Geometry check sheet. Reference: the model listing, model coordinates, mm. A direction names the side the tool comes from. Coordinates: 2 decimals unless noted, no trailing zeros. Write each loop counter-clockwise with the first axis right and the second up, starting at its lowest first coordinate (ties: lowest second). Pieces come first, ordered by that corner, then holes. Notation, with made-up numbers: (64, 83) -> (100, 83) arc R13 ccw to (100, 100) -> close; hole circle Ø10 at (68, -7). An arc over 180 degrees is marked (long way). Put each result on its own line as item: value. Start each with the question number.
from build123d import *

# Parameters (mm, degrees)
SKETCH_1_W          = 280
SKETCH_1_H          = 230
EXTRUDE_1_DEPTH     = 2
SKETCH_2_R          = 2.15
CUT_EXTRUDE_1_DEPTH = 182.18774793
SKETCH_3_R          = 30
CUT_EXTRUDE_2_DEPTH = 182.18774793
SKETCH_4_R          = 1.6
CUT_EXTRUDE_3_DEPTH = 182.18774793
SKETCH_5_R          = 1.65
CUT_EXTRUDE_4_DEPTH = 182.18774793
SKETCH_7_W          = 25
SKETCH_7_H          = 115
SKETCH_7_W_2        = 85
SKETCH_7_H_2        = 15
CUT_EXTRUDE_5_DEPTH = 182.18774793
SKETCH_9_W          = 36
SKETCH_9_H          = 17
CUT_EXTRUDE_6_DEPTH = 182.18774793
FILLET_1_R          = 2
FILLET_2_R          = 2


with BuildPart() as part:
    # 草图1 → 凸台-拉伸1 (new body)
    with BuildSketch(Plane.XY):
        Rectangle(SKETCH_1_W, SKETCH_1_H)
    extrude(amount=EXTRUDE_1_DEPTH)

    # 草图2 → 切除-拉伸1 (cut, through all)
    with BuildSketch(Plane.XY.offset(2)):
        with Locations((-132.5, -105)):
            Circle(SKETCH_2_R)
        with Locations(Location((132.5, -105, 0), (0, 0, 180))):
            Circle(SKETCH_2_R)
        with Locations((-115, -87.5)):
            Circle(SKETCH_2_R)
        with Locations((-95, -87.5)):
            Circle(SKETCH_2_R)
        with Locations((-75, -87.5)):
            Circle(SKETCH_2_R)
        with Locations(Location((75, -87.5, 0), (0, 0, 180))):
            Circle(SKETCH_2_R)
        with Locations(Location((95, -87.5, 0), (0, 0, 180))):
            Circle(SKETCH_2_R)
        with Locations(Location((115, -87.5, 0), (0, 0, 180))):
            Circle(SKETCH_2_R)
    extrude(amount=-CUT_EXTRUDE_1_DEPTH, mode=Mode.SUBTRACT)

    # 草图3 → 切除-拉伸2 (cut, through all)
    with BuildSketch(Plane.XY.offset(2)):
        with Locations((0, -5)):
            Circle(SKETCH_3_R)
        with BuildLine():
            ThreePointArc((30, -5), (0, -35), (-30, -5))
            Line((-30, -5), (-30, -115))
            Line((-30, -115), (30, -115))
            Line((30, -115), (30, -5))
        make_face()
    extrude(amount=-CUT_EXTRUDE_2_DEPTH, mode=Mode.SUBTRACT)

    # 草图4 → 切除-拉伸3 (cut, through all)
    with BuildSketch(Plane.XY.offset(2)):
        with Locations((-109, -35)):
            Circle(SKETCH_4_R)
        with Locations((-109, -55)):
            Circle(SKETCH_4_R)
        with Locations((-116, -35)):
            Circle(SKETCH_4_R)
        with Locations((-116, -55)):
            Circle(SKETCH_4_R)
        with Locations(Location((116, -55, 0), (0, 0, 180))):
            Circle(SKETCH_4_R)
        with Locations(Location((116, -35, 0), (0, 0, 180))):
            Circle(SKETCH_4_R)
        with Locations(Location((109, -55, 0), (0, 0, 180))):
            Circle(SKETCH_4_R)
        with Locations(Location((109, -35, 0), (0, 0, 180))):
            Circle(SKETCH_4_R)
    extrude(amount=-CUT_EXTRUDE_3_DEPTH, mode=Mode.SUBTRACT)

    # 草图5 → 切除-拉伸4 (cut, through all)
    with BuildSketch(Plane.XY.offset(2)):
        with Locations((-60, 109)):
            Circle(SKETCH_5_R)
        with Locations((-80, 109)):
            Circle(SKETCH_5_R)
        with Locations(Location((80, 109, 0), (0, 0, 180))):
            Circle(SKETCH_5_R)
        with Locations(Location((60, 109, 0), (0, 0, 180))):
            Circle(SKETCH_5_R)
    extrude(amount=-CUT_EXTRUDE_4_DEPTH, mode=Mode.SUBTRACT)

    # 草图7 → 切除-拉伸5 (cut, through all)
    with BuildSketch(Plane.XY.offset(2)):
        Polygon((-90, 69), (-90, -69), (-59.885931147, 0), align=None)
        Polygon((-90, 94), (-66.432467855, 40), (66.432467855, 40), (90, 94), align=None)
        Polygon((-40, 20.564392374), (-79.089105488, -69), (-40, -69), align=None)
        Polygon((40, -69), (40, 20.564392374), (79.089105488, -69), align=None)
        Polygon((59.885931147, 0), (90, 69), (90, -69), align=None)
        with Locations((112.5, 36.5)):
            Rectangle(SKETCH_7_W, SKETCH_7_H)
        with Locations((-112.5, 36.5)):
            Rectangle(SKETCH_7_W, SKETCH_7_H)
        with Locations((72.5, -107.5)):
            Rectangle(SKETCH_7_W_2, SKETCH_7_H_2)
        with Locations((-72.5, -107.5)):
            Rectangle(SKETCH_7_W_2, SKETCH_7_H_2)
    extrude(amount=-CUT_EXTRUDE_5_DEPTH, mode=Mode.SUBTRACT)

    # 草图9 → 切除-拉伸6 (cut, through all)
    with BuildSketch(Plane.XY.offset(2)):
        with Locations((48, -91.5)):
            Rectangle(SKETCH_9_W, SKETCH_9_H)
        with Locations((-48, -91.5)):
            Rectangle(SKETCH_9_W, SKETCH_9_H)
    extrude(amount=-CUT_EXTRUDE_6_DEPTH, mode=Mode.SUBTRACT)

    # 圆角1
    fillet_1_edges = [part.edges().sort_by_distance(p)[0] for p in [
        (79.089105488, -69, 1),
        (40, -69, 1),
        (40, 20.564392374, 1),
        (-40, -69, 1),
        (-79.089105488, -69, 1),
        (-40, 20.564392374, 1),
        (66.432467855, 40, 1),
        (-66.432467855, 40, 1),
        (-90, 94, 1),
        (90, 94, 1),
        (-125, -21, 1),
        (-125, 94, 1),
        (-100, 94, 1),
        (-100, -21, 1),
        (90, -69, 1),
        (59.885931147, 0, 1),
        (90, 69, 1),
        (100, 94, 1),
        (125, 94, 1),
        (125, -21, 1),
        (100, -21, 1),
        (-90, 69, 1),
        (-59.885931147, 0, 1),
        (-90, -69, 1),
    ]]
    fillet(fillet_1_edges, radius=FILLET_1_R)

    # 圆角2
    fillet_2_edges = [part.edges().sort_by_distance(p)[0] for p in [
        (115, -115, 1),
        (115, -100, 1),
        (-115, -115, 1),
        (-115, -100, 1),
        (-30, -83, 1),
        (-66, -100, 1),
        (-66, -83, 1),
        (66, -100, 1),
        (30, -83, 1),
        (66, -83, 1),
        (140, -115, 1),
        (-140, -115, 1),
        (-140, 115, 1),
        (140, 115, 1),
    ]]
    fillet(fillet_2_edges, radius=FILLET_2_R)


solid = part.part
Item 1: Section check C-C, the plane x = -50. Enter the section's corners in (y, z).
Item 2: Go/stop test with flat-tipped pins: P1, Ø6, axis at x = -82.5, y = -39, coming from the +Z side; P2, Ø1, axis at x = -80.5, z = 1.5, coming from the -Y side; P3, Ø0.6, axis at x = 6.5, z = 1, coming from the -Y side; P4, Ø1, axis at x = 113.5, z = 1.5, coming from the -Y side. Record where each tip stops, or that it passes through.
Item 3: Scan lines: line 1 along X through (y, z) = (109, 0.8); line 2 along X through (y, z) = (50.5, 0.3); line 3 along Y through (x, z) = (-60, 1.3). Record each from-to range of solid material in increasing order. Write a range as [from, to].
Item 4: Section check A-A, the plane x = 0. Enter the section's corners in (y, z), and give its area (3 significant figures).
Item 5: Section check B-B, the plane y = 5.5. Give the number of separate pieces and of enclosed holes in the cut face, and give its area (3 significant figures).
Item 6: Access from +Z, -Z, +X, -X, +Y, -Y to the whole of each face (thin tool, end or side, straight path). Record for faces 1 (the flat face through (-60.61, -26.66, 1.01)), 2 (the flat face through (-33, 2, 0)).
Item 7: Mould release check, pull along Y, two halves, no side actions. Record for faces 3 (the flat face through (-33, 2, 2)), 4 (the flat face through (77.714, 65.85, 1.014)), 5 (the cylindrical face through (0.66, 24.993, 1.014)): released by +Y, released by -Y, zero draft, split by the parting line, or undercut.
From the geometry:
1. outline: (-83, 0) -> (-69, 0) -> (-69, 2) -> (-83, 2) -> close; (-2.35, 0) -> (40, 0) -> (40, 2) -> (-2.35, 2) -> close; (94, 0) -> (115, 0) -> (115, 2) -> (94, 2) -> close
2. P1: through
2. P2: y = -100
2. P3: y = 24.22
2. P4: y = -100.27
3. line 1: [-140, -81.65], [-78.35, -61.65], [-58.35, 58.35], [61.65, 78.35], [81.65, 140]
3. line 2: [-140, -125], [-100, -90], [-81.93, -71.02], [71.02, 81.93], [90, 100], [125, 140]
3. line 3: [-83, -69], [-25.26, 40], [94, 107.35], [110.65, 115]
4. outline: (25, 0) -> (40, 0) -> (40, 2) -> (25, 2) -> close; (94, 0) -> (115, 0) -> (115, 2) -> (94, 2) -> close
4. area: 72.0 mm²
5. separate pieces: 8
5. enclosed holes: 0
5. area: 210 mm²
6. face 1: +Z, -Z
6. face 2: -Z, +X, -X, +Y, -Y
7. face 3: zero draft
7. face 4: undercut
7. face 5: released by -Y
